Check sheet for the modelled part. Datum: model origin and axes. Units: mm. Round coordinates to 2 decimals unless told otherwise and drop trailing zeros. Write each loop counter-clockwise with the first axis right and the second up, starting at its lowest first coordinate (ties: lowest second). Pieces come first, ordered by that corner, then holes. Notation, with made-up numbers: (5, -34.75) -> (30, -34.75) arc R33 cw to (30, -3.75) -> close; hole circle Ø6 at (6, 54). An arc over 180 degrees is marked (long way). Write item = value, one per line.
from build123d import *

# Parameters (mm, degrees)
F0_W     = 200
F0_H     = 200
F1_DEPTH = 20
F2_R     = 3.75
F3_DEPTH = 30


with BuildPart() as f1:
    # F0 (on Front) → F1 (new body)
    with BuildSketch(Plane.XZ):
        Rectangle(F0_W, F0_H)
    extrude(amount=F1_DEPTH)

    # F2 (on face) → F3 (join)
    with BuildSketch(Plane.XZ.offset(20)):
        with Locations((-40, 53.214375)):
            Circle(F2_R)
        with Locations((-22, 53.214375)):
            Circle(F2_R)
        with Locations((-22, 33.214375)):
            Circle(F2_R)
        with Locations((0, 33.214375)):
            Circle(F2_R)
        with Locations((0, 9.214375)):
            Circle(F2_R)
        with Locations((0, -16.785625)):
            Circle(F2_R)
        with Locations((0, -44.785625)):
            Circle(F2_R)
    extrude(amount=F3_DEPTH)


solid = f1.part
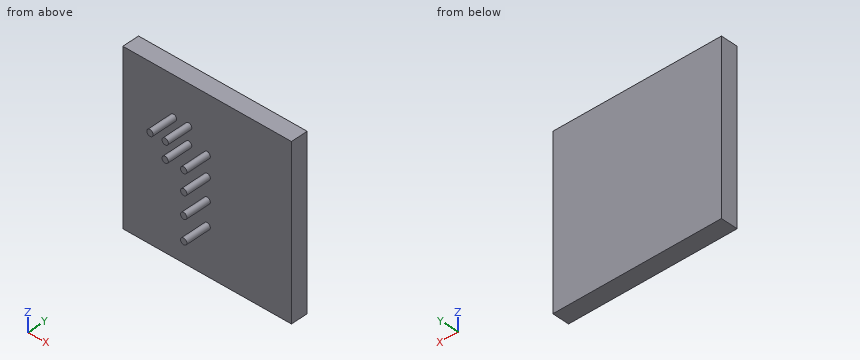
(1) Sectioned sample at A-A on x = -22. Enter the section's corners in (y, z).
Worked answers:
outline = (-50, 29.46) -> (-20, 29.46) -> (-20, -100) -> (0, -100) -> (0, 100) -> (-20, 100) -> (-20, 56.96) -> (-50, 56.96) -> (-50, 49.46) -> (-20, 49.46) -> (-20, 36.96) -> (-50, 36.96) -> close
(2) Go/stop test with flat-tipped pins: P1, Ø2, axis at x = -3, z = -41, coming from the -Y side; P2, Ø12, axis at x = 16.5, z = 5.5, coming from the +Y side; P3, Ø8, axis at y = -33.5, z = -10.5, coming from the +X side; P4, Ø5, axis at y = -29.5, z = -45, coming from the +X side. Record where each tip stops, or that it passes through.
Worked answers:
P1 = -20
P2 = 0
P3 = 2.97
P4 = 3.75
(3) Material ranges on L1, parallel to Y at x = -81.5, z = -40.5; L2, parallel to X at y = -35, z = 56.5; L3, parallel to Z at x = -42.5, y = -39, recorded low to high. Write a range as [from, to].
Worked answers:
L1 = [-20, 0]
L2 = [-41.81, -38.19], [-23.81, -20.19]
L3 = [50.42, 56.01]
(4) Sectioned sample at D-D on x = 0. Enter the section's corners in (y, z).
Worked answers:
outline = (-50, -48.54) -> (-20, -48.54) -> (-20, -100) -> (0, -100) -> (0, 100) -> (-20, 100) -> (-20, 36.96) -> (-50, 36.96) -> (-50, 29.46) -> (-20, 29.46) -> (-20, 12.96) -> (-50, 12.96) -> (-50, 5.46) -> (-20, 5.46) -> (-20, -13.04) -> (-50, -13.04) -> (-50, -20.54) -> (-20, -20.54) -> (-20, -41.04) -> (-50, -41.04) -> close
(5) Sectioned sample at B-B on y = -35. Enter the section's corners in (x, z).
Worked answers:
outline = circle Ø7.5 at (-40, 53.21); circle Ø7.5 at (-22, 33.21); circle Ø7.5 at (-22, 53.21); circle Ø7.5 at (0, -44.79); circle Ø7.5 at (0, -16.79); circle Ø7.5 at (0, 9.21); circle Ø7.5 at (0, 33.21)
(6) Sectioned sample at C-C on z = 16. Enter the section's corners in (x, y), then the cut area to 3 significant figures.
Worked answers:
outline = (-100, -20) -> (100, -20) -> (100, 0) -> (-100, 0) -> close
area = 4,000 mm²
